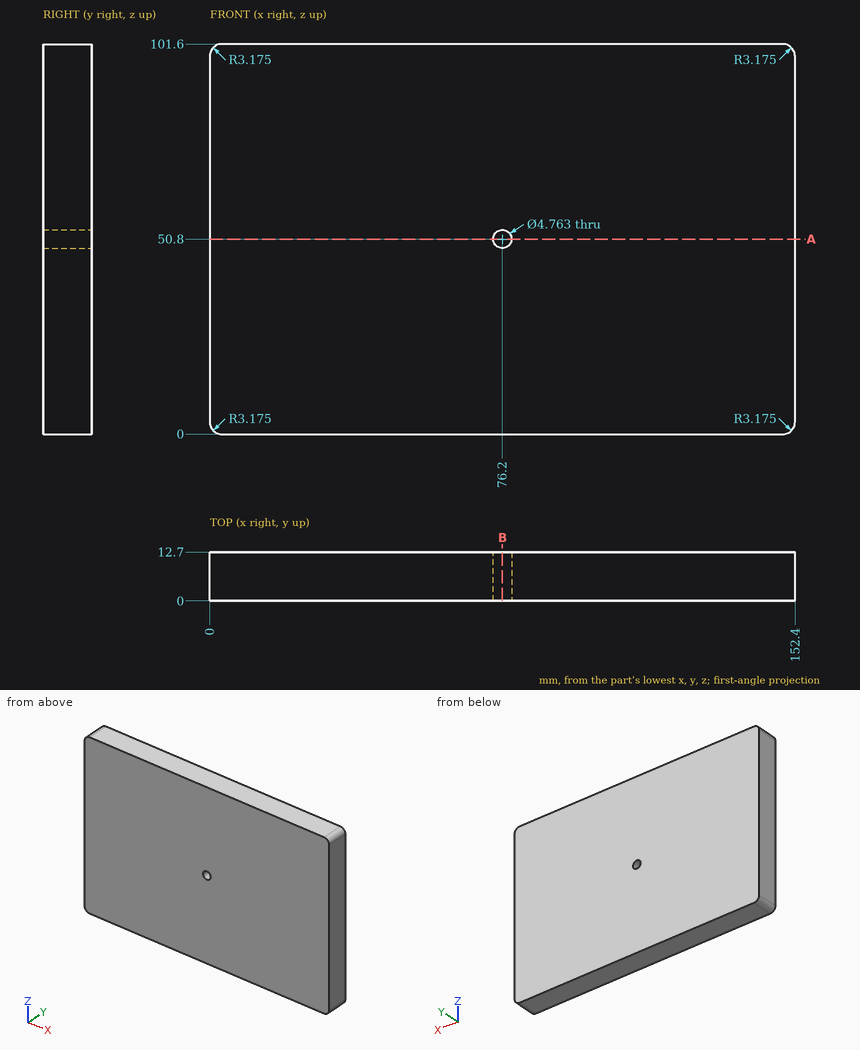
Here's the drawing with two shaded views (mm, measured from the low corner). I have some questions. Give positions to 0.01 mm unless a question says otherwise; leave off trailing zeros. Loops run counter-clockwise (first coordinate to the right, second up) from the corner with the lowest first, then second, coordinate; pieces in that order, holes last. Notation, with made-up numbers: (-21, -27.75) -> (18, -27.75) arc R26 cw to (18, -7.75) -> close; hole circle Ø10 at (48.5, -30). An arc over 180 degrees is marked (long way). Answer as a JSON object with one key per item and string values. Group by question number.
Item 1: Imagine slicing it at A-A on z = 50.8. Write out the boundary of the cut face in (x, y), then the cut area to 4 significant figures.
Item 2: I need wall thicknesses on L1, parallel to Z at x = 76.2, y = 4.5; L2, parallel to X at y = 4.5, z = 50.8. Which ranges of each line are inside material? Lowest first, please.
Item 3: Imagine slicing it at B-B on x = 76.2. Write out the boundary of the cut face in (y, z).
Answer list:
{
 "1": {"outline": "(0, 0) -> (73.82, 0) -> (73.82, 12.7) -> (0, 12.7) -> close; (78.58, 0) -> (152.4, 0) -> (152.4, 12.7) -> (78.58, 12.7) -> close", "area": "1,875 mm2"},
 "2": {"L1": "z = 0 to 48.42, 53.18 to 101.6", "L2": "x = 0 to 73.82, 78.58 to 152.4"},
 "3": {"outline": "(0, 0) -> (12.7, 0) -> (12.7, 48.42) -> (0, 48.42) -> close; (0, 53.18) -> (12.7, 53.18) -> (12.7, 101.6) -> (0, 101.6) -> close"}
}
